```python
from build123d import *

# Parameters (mm, degrees)
F1_DEPTH = 2.2


with BuildPart() as f1:
    # F0 (on Top) → F1 (new body)
    with BuildSketch(Plane.XY):
        with BuildLine():
            ThreePointArc((0, 6), (1.757359, 1.757359), (6, 0))
            Line((6, 0), (20, 0))
            ThreePointArc((20, 0), (24.242641, 1.757359), (26, 6))
            Line((26, 6), (26, 30.880977))
            ThreePointArc((26, 30.880977), (24.797058, 34.13403), (21.76706, 35.821789))
            ThreePointArc((21.76706, 35.821789), (13, 36.498279), (4.23294, 35.821789))
            ThreePointArc((4.23294, 35.821789), (1.202942, 34.13403), (0, 30.880977))
            Line((0, 30.880977), (0, 6))
        make_face()
        with BuildLine():
            ThreePointArc((6, 27), (6.585786, 28.414214), (8, 29))
            Line((8, 29), (18, 29))
            ThreePointArc((18, 29), (19.414214, 28.414214), (20, 27))
            Line((20, 27), (20, 16))
            ThreePointArc((20, 16), (18.242641, 11.757359), (14, 10))
            Line((14, 10), (12, 10))
            ThreePointArc((12, 10), (7.757359, 11.757359), (6, 16))
            Line((6, 16), (6, 27))
        make_face(mode=Mode.SUBTRACT)
    extrude(amount=F1_DEPTH)


solid = f1.part
```
For this review, take the finished solid that the model builds, in its own axes (mm). A direction names the side the tool comes from. Give positions to 0.01 mm unless a question says otherwise; leave off trailing zeros. Order: outer loops, then holes, each group sorted by start corner. A loop starts at its lowest first (then second) coordinate and runs counter-clockwise, first axis right, second up.
1) Insertion check: pin 1 (1 mm diameter, centred on x = 4.5, z = 0.5, fed in from -Y); pin 2 (0.6 mm diameter, centred on x = 12.5, z = 1.5, fed in from +Y). Each pin has a flat end and moves straight along its axis. Give the tip position at first contact, or say it passes through.
2) Take a section at C-C (x = 13.5). Give the boundary of the cut face in (y, z), then the cut area to 3 significant figures.
3) Take a section at D-D (x = 23.5). Give the boundary of the cut face in (y, z).
4) For faces 4 (the face through (21, 19, 0)), 5 (the face through (6.57, 28.4, 1.08)), list the 3-axis set-ups (+Z, -Z, +X, -X, +Y, -Y) from which the entire face can be reached by the end or side of a thin tool; tool diameter is ignored.
5) Take a section at A-A (z = 1.1). Give the boundary of the cut face in (x, y), then the cut area to 3 significant figures.
6) Wall thickness on line 1 (X direction, y = 22, z = 1); line 2 (Y direction, x = 17, z = 0.45); line 3 (Y direction, x = 11.5, z = 1.2): over which ranges is each line inside the solid? List them lowest first.
7) The part is to be moulded in two halves that separate along Y. For faces 1 (the face through (0, 19, 1)), 2 (the face through (24.196, 1.711, 1.085)), 3 (the face through (13, 29, 1)), say which applies: released by +Y, released by -Y, zero draft, split by the parting line, or undercut.
8) Take a section at B-B (y = 20). Give the boundary of the cut face in (x, z).
Derived:
1. pin 1: stops at y = 0.08
1. pin 2: stops at y = 36.5
2. outline: (0, 0) - (10, 0) - (10, 2.2) - (0, 2.2) - close; (29, 0) - (36.5, 0) - (36.5, 2.2) - (29, 2.2) - close
2. area: 38.5 mm2
3. outline: (1.13, 0) - (35.21, 0) - (35.21, 2.2) - (1.13, 2.2) - close
4. face 4: -Z, +X, -X, +Y, -Y
4. face 5: +Z, -Z
5. outline: (0, 6) arc R6 ccw to (6, 0) - (20, 0) arc R6 ccw to (26, 6) - (26, 30.88) arc R5 ccw to (21.77, 35.82) arc R57.15 ccw to (4.23, 35.82) arc R5 ccw to (0, 30.88) - close; hole (6, 16) arc R6 ccw to (12, 10) - (14, 10) arc R6 ccw to (20, 16) - (20, 27) arc R2 ccw to (18, 29) - (8, 29) arc R2 ccw to (6, 27) - close
5. area: 665 mm2
6. line 1: x = 0 to 6, 20 to 26
6. line 2: y = 0 to 10.8, 29 to 36.36
6. line 3: y = 0 to 10.02, 29 to 36.48
7. face 1: zero draft
7. face 2: released by -Y
7. face 3: undercut
8. outline: (0, 0) - (6, 0) - (6, 2.2) - (0, 2.2) - close; (20, 0) - (26, 0) - (26, 2.2) - (20, 2.2) - close
